Can you work these out from the model? Positions are in its coordinate system, mm. Face numbers are marked on the shaded views. A direction names the side the tool comes from. Round coordinates to 2 decimals unless told otherwise and drop trailing zeros. Loops run counter-clockwise (first coordinate to the right, second up) from the corner with the lowest first, then second, coordinate; pieces in that order, holes last. Notation, with made-up numbers: (56, 9.25) -> (77, 9.25) arc R13 cw to (77, 24.25) -> close; hole circle Ø3 at (41.5, -6.5). An arc over 180 degrees is marked (long way). Answer as a JSON object with one key per item and string values.
```python
from build123d import *

# Parameters (mm, degrees)
PAD_DEPTH         = 6
SKETCH001_W       = 8
SKETCH001_H       = 20
PAD001_DEPTH      = 25
PAD001_DEPTH_BACK = 4
SKETCH002_W       = 17.981461
SKETCH002_H       = 19.878344
POCKET_DEPTH      = 6
SKETCH003_R       = 2.6
POCKET001_DEPTH   = 9
FILLET_R          = 3


with BuildPart() as part:
    # Sketch → Pad (new body)
    with BuildSketch(Plane.XY):
        Polygon((62, 42), (62, 0), (10, 0), (0, 0), (0, 42), align=None)
        with BuildLine():
            ThreePointArc((16, 38.6), (14.4, 37), (16, 35.4))
            Line((16, 35.4), (24, 35.4))
            ThreePointArc((24, 35.4), (25.6, 37), (24, 38.6))
            Line((16, 38.6), (24, 38.6))
        make_face(mode=Mode.SUBTRACT)
        with BuildLine():
            Line((47, 38.6), (55, 38.6))
            ThreePointArc((55, 35.4), (56.6, 37), (55, 38.6))
            Line((47, 35.4), (55, 35.4))
            ThreePointArc((47, 38.6), (45.4, 37), (47, 35.4))
        make_face(mode=Mode.SUBTRACT)
        with BuildLine():
            ThreePointArc((16, 7.6), (14.4, 6), (16, 4.4))
            Line((16, 4.4), (24, 4.4))
            ThreePointArc((24, 4.4), (25.6, 6), (24, 7.6))
            Line((16, 7.6), (24, 7.6))
        make_face(mode=Mode.SUBTRACT)
        with BuildLine():
            ThreePointArc((48, 7.6), (46.4, 6), (48, 4.4))
            Line((48, 4.4), (56, 4.4))
            ThreePointArc((56, 4.4), (57.6, 6), (56, 7.6))
            Line((48, 7.6), (56, 7.6))
        make_face(mode=Mode.SUBTRACT)
        with BuildLine():
            ThreePointArc((31, 32.75), (19.25, 21), (31, 9.25))
            Line((31, 9.25), (41, 9.25))
            ThreePointArc((41, 9.25), (52.75, 21), (41, 32.75))
            Line((31, 32.75), (41, 32.75))
        make_face(mode=Mode.SUBTRACT)
    extrude(amount=PAD_DEPTH)

    # Sketch001 (on Face27 of Pad) → Pad001 (join, two sides)
    with BuildSketch(Plane.XY.offset(6)) as pad001_sk:
        with Locations((4, 21.25)):
            Rectangle(SKETCH001_W, SKETCH001_H)
    extrude(amount=PAD001_DEPTH)
    extrude(pad001_sk.sketch, amount=-PAD001_DEPTH_BACK)

    # Sketch002 (on Face5 of Pad001) → Pocket (cut)
    with BuildSketch(Plane.XY.offset(6)):
        with Locations((16.99073, 21.310828)):
            Rectangle(SKETCH002_W, SKETCH002_H)
    extrude(amount=-POCKET_DEPTH, mode=Mode.SUBTRACT)

    # Sketch003 (on Face34 of Pocket) → Pocket001 (cut)
    with BuildSketch(Plane.YZ.offset(8)):
        with Locations((21.119102, 26)):
            Circle(SKETCH003_R)
        with Locations((21.393444, 6)):
            Circle(SKETCH003_R)
    extrude(amount=-POCKET001_DEPTH, mode=Mode.SUBTRACT)

    # Fillet
    fillet_edges = [part.edges().sort_by_distance(p)[0] for p in [
        (0, 0, 3),
        (62, 0, 3),
        (62, 42, 3),
        (0, 42, 3),
        (4, 31.25, 31),
        (4, 11.25, 31),
    ]]
    fillet(fillet_edges, radius=FILLET_R)


solid = part.part
```
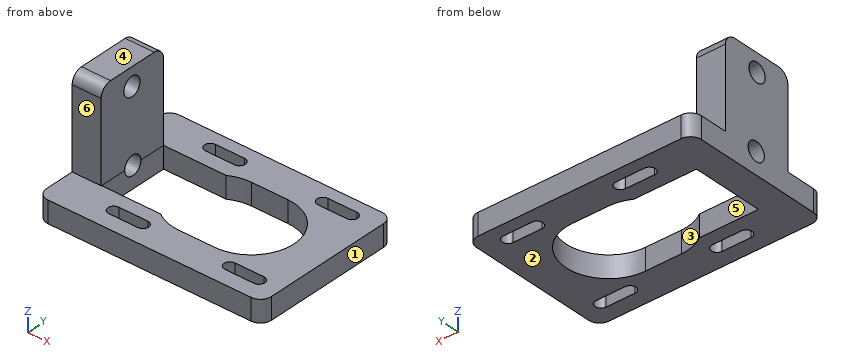
Q1. I want a section at B-B, the plane x = 20.5. Write out the boundary of the cut face in (y, z), then the cut area to 3 significant figures.
Determined:
{"outline": "(0, 0) -> (4.4, 0) -> (4.4, 6) -> (0, 6) -> close; (7.6, 0) -> (11.37, 0) -> (11.37, 6) -> (7.6, 6) -> close; (31.25, 0) -> (35.4, 0) -> (35.4, 6) -> (31.25, 6) -> close; (38.6, 0) -> (42, 0) -> (42, 6) -> (38.6, 6) -> close", "area": "94.3 mm²"}
Q2. I want a section at C-C, the plane x = 33.5. Write out the boundary of the cut face in (y, z), then the cut area to 3 significant figures.
Determined:
{"outline": "(0, 0) -> (9.25, 0) -> (9.25, 6) -> (0, 6) -> close; (32.75, 0) -> (42, 0) -> (42, 6) -> (32.75, 6) -> close", "area": "111 mm²"}
Q3. I want a section at A-A, the plane y = 6. Write out the boundary of the cut face in (x, z), then the cut area to 3 significant figures.
Determined:
{"outline": "(0, 0) -> (14.4, 0) -> (14.4, 6) -> (0, 6) -> close; (25.6, 0) -> (46.4, 0) -> (46.4, 6) -> (25.6, 6) -> close; (57.6, 0) -> (62, 0) -> (62, 6) -> (57.6, 6) -> close", "area": "238 mm²"}
Q4. We'd pull the mould along X, two halves only. Please class the marked faces 1, 2 and 3: pulls with the +X half, pulls with the -X half, needs draft (parallel to the pull), parting line crosses it, or undercut.
Determined:
{"face 1": "pulls with the +X half", "face 2": "needs draft", "face 3": "undercut"}
Q5. I want a section at D-D, the plane z = 2.5. Give the number of separate pieces and of enclosed holes in the cut face, then the cut area to 3 significant figures.
Determined:
{"separate pieces": "1", "enclosed holes": "5", "area": "1,540 mm²"}
Q6. On a 3-axis mill with a long thin cutter (end or side, diameter ignored), from which of +Z, -Z, +X, -X, +Y, -Y can I reach the whole of each face in a straight line? I mean the marked faces 4, 5 and 6. Say none if no direction works.
Determined:
{"face 4": "+Z, +X, -X, +Y, -Y", "face 5": "+Z, -Z", "face 6": "+Z, +X, -X, -Y"}
Q7. If I drill on L1, parallel to X at y = 27, z = 27; L2, parallel to Z at x = 44, y = 40; L3, parallel to X at y = 30, z = 1, over which ranges is the centre line in solid material (lowest first)? Write a range as [from, to].
Determined:
{"L1": "[0, 8]", "L2": "[0, 6]", "L3": "[0, 8], [48.55, 62]"}
Q8. I'm going to push flat-ended pins straight in: pin 1 (6.5 mm diameter, centred on x = 2.5, z = 19.5, fed in from +Y); pin 2 (1.5 mm diameter, centred on x = 56, y = 25.5, fed in from +Z); pin 3 (4 mm diameter, centred on x = 2.5, z = 13, fed in from -Y). Where does each tip first touch, or does it pass through?
Determined:
{"pin 1": "y = 31.25", "pin 2": "z = 6", "pin 3": "y = 11.25"}
